Autodesk Inventor part; units mm, degrees
ref_plane "YZ Plane" through (0, 0, 0) normal (1, 0, 0) x (0, 1, 0)
ref_plane "XZ Plane" through (0, 0, 0) normal (0, 1, 0) x (-1, 0, 0)
ref_plane "XY Plane" through (0, 0, 0) normal (0, 0, 1) x (1, 0, 0)
sketch "Sketch1" plane through (0, 0, 0) normal (0, 1, 0) x (-1, 0, 0)
  line L0 (15.8302, -38.0798) -> (-15.7328, -38.1201)
  line L1 (-15.7328, -38.1201) -> (-38.0798, -15.8302)
  line L2 (-38.0798, -15.8302) -> (-38.1201, 15.7328)
  line L3 (-38.1201, 15.7328) -> (-15.8302, 38.0798)
  line L4 (-15.8302, 38.0798) -> (15.7328, 38.1201)
  line L5 (15.7328, 38.1201) -> (38.0798, 15.8302)
  line L6 (38.0798, 15.8302) -> (38.1201, -15.7328)
  line L7 (38.1201, -15.7328) -> (15.8302, -38.0798)
  point P0 (0, 0)
  point P1 (0, 0)
  dimension "d0" = 76.2
extrude "Extrusion1" add sketch "Sketch1" along normal blind 3.175
sketch "Sketch3" plane through (0, 3.175, 0) normal (0, 1, 0) x (1, 0, 0)
  line L0 (38.1201, -15.7328) -> (38.0798, 15.8302)
  line L1 (-38.1201, 15.7328) -> (-38.0798, -15.8302)
  line L2 (32.9198, -20.9465) -> (32.8661, 21.0306)
  line L3 (-32.9198, 20.9465) -> (-32.8661, -21.0306)
  line L4 (-38.1201, 15.7328) -> (-38.0798, -15.8302)
  line L5 (38.1201, -15.7328) -> (38.0798, 15.8302)
  line L6 (38.1201, -15.7328) -> (32.9198, -20.9465)
  line L7 (38.0798, 15.8302) -> (38.1201, -15.7328)
  line L8 (38.1201, -15.7328) -> (38.0798, 15.8302)
  line L9 (38.0798, 15.8302) -> (32.8661, 21.0306)
  line L10 (-32.9198, 20.9465) -> (-38.1201, 15.7328)
  line L11 (-38.1201, 15.7328) -> (-38.0798, -15.8302)
  line L12 (-38.0798, -15.8302) -> (-38.1201, 15.7328)
  line L13 (-38.0798, -15.8302) -> (-32.8661, -21.0306)
  line L14 (-38.0798, -15.8302) -> (-15.7328, -38.1201)
  line L15 (15.8302, -38.0798) -> (38.1201, -15.7328)
  line L16 (38.0798, 15.8302) -> (15.7328, 38.1201)
  line L17 (38.1201, -15.7328) -> (32.9198, -20.9465)
  line L18 (38.0798, 15.8302) -> (32.8661, 21.0306)
  line L19 (15.7328, 38.1201) -> (38.0798, 15.8302)
  line L20 (38.1201, -15.7328) -> (38.0798, 15.8302)
  point P0 (0, 0)
  dimension "d5" = 5.207
  dimension "d6" = 5.207
extrude "Extrusion2" add sketch "Sketch3" along normal blind 35.56
sketch "Sketch5" plane through (38.0798, 0, -15.8302) normal (1, 0, -0.0013) x (-0.0013, 0, -1)
  circle A0 centre (-15.7815, 18.415) radius 11.43
  circle A1 centre (-15.7815, 18.415) radius 11.684
  point P0 (-15.7815, 0)
  dimension "d9" = 0.254
extrude "Extrusion3" cut sketch "Sketch5" against normal blind 26.416 contours A0 | A1
sketch "Sketch6" plane through (-38.0798, 0, 15.8302) normal (-1, 0, 0.0013) x (0.0013, 0, 1)
  circle A0 centre (-15.7815, 18.415) radius 11.43
  circle A1 centre (-15.7815, 18.415) radius 11.684
  point P0 (-15.7815, 0)
  dimension "d12" = 0.254
extrude "Extrusion4" cut sketch "Sketch6" against normal blind 26.416 contours A0 | A1
sketch "Sketch7" plane through (0, 3.175, 0) normal (0, 1, 0) x (1, 0, 0)
  line L0 (15.7328, 38.1201) -> (-15.8302, 38.0798)
  line L1 (20.9465, 32.9198) -> (-21.0306, 32.8661)
  line L2 (-15.8302, 38.0798) -> (-32.9198, 20.9465)
  line L3 (32.8661, 21.0306) -> (15.7328, 38.1201)
  line L4 (-38.1201, 15.7328) -> (-15.8302, 38.0798)
  line L5 (-21.0306, 32.8661) -> (-15.8302, 38.0798)
  line L6 (-15.8302, 38.0798) -> (15.7328, 38.1201)
  line L7 (20.9465, 32.9198) -> (15.7328, 38.1201)
  point P0 (0, 0)
  dimension "d15" = 5.207
extrude "Extrusion5" add sketch "Sketch7" along normal blind 35.56
sketch "Sketch8" plane through (-15.8302, 0, -38.0798) normal (-0.0013, 0, -1) x (-1, 0, 0.0013)
  circle A0 centre (-15.7815, 18.415) radius 11.43
  circle A1 centre (-15.7815, 18.415) radius 11.684
  point P0 (-15.7815, 0)
  dimension "d18" = 0.254
extrude "Extrusion6" cut sketch "Sketch8" against normal blind 26.416 contours A0 | A1
sketch "Sketch9" plane through (0, 3.175, 0) normal (0, 1, 0) x (1, 0, 0)
  line L0 (-9.3728, -20.3542) -> (-9.3647, -26.7042)
  line L1 (8.6353, -26.6812) -> (8.6272, -20.3312)
  line L2 (-8.3634, -27.7029) -> (7.6366, -27.6825)
  line L3 (-9.3728, -20.3542) -> (8.6366, -20.3542)
  line L4 (8.6366, -20.3542) -> (8.6366, -27.6812)
  line L5 (8.6366, -27.6812) -> (-9.3728, -27.6812)
  line L6 (-9.3728, -27.6812) -> (-9.3728, -20.3542)
  point P0 (0, 0)
extrude "Extrusion7" add sketch "Sketch9" along normal blind 26.67
sketch "Sketch10" plane through (0, 29.845, 0) normal (0, 1, 0) x (1, 0, 0)
  arc A0 (-5.3692, -23.1491) -> (-5.3658, -25.8491) centre (-5.3675, -24.4991) ccw
  arc A1 (-5.3658, -25.8491) -> (-5.3692, -23.1491) centre (-5.3675, -24.4991) ccw
  arc A2 (4.6308, -23.1363) -> (4.6342, -25.8363) centre (4.6325, -24.4863) ccw
  arc A3 (4.6342, -25.8363) -> (4.6308, -23.1363) centre (4.6325, -24.4863) ccw
  circle A4 centre (-5.3675, -24.4991) radius 1.016
  circle A5 centre (4.6325, -24.4863) radius 1.016
  point P0 (0, 0)
  dimension "d24" = 1.35
  dimension "d25" = 2.032
  dimension "d26" = 2.032
extrude "Extrusion8" cut sketch "Sketch10" against normal blind 12.7 contours A4 | A5
sketch "Sketch11" plane through (-9.3728, 3.175, 27.6812) normal (0, 0, 1) x (1, 0, 0)
  line L0 (18.0094, 0) -> (0, 0)
  line L1 (5.1947, 6.35) -> (12.8147, 6.35)
  line L2 (12.8147, 6.35) -> (12.8147, 0)
  line L3 (12.8147, 0) -> (5.1947, 0)
  line L4 (5.1947, 0) -> (5.1947, 6.35)
  line L5 (18.0094, 0) -> (18.0094, 26.67)
  point P0 (9.3728, -3.175)
  dimension "d31" = 5.1947
  dimension "d32" = 7.62
  dimension "d33" = 6.35
  dimension "d36" = 0
extrude "Extrusion9" cut sketch "Sketch11" against normal blind 12.7
fillet "Fillet2" radius 3.175 4 edges at (-6.7754, 3.175, 27.6812) (-9.3728, 3.175, 24.0177) (6.0392, 3.175, 27.6812) (8.6366, 3.175, 24.0177)
properties part number "Main_assy_base"
For this review, take the finished solid that the model builds, in its own axes (mm). Give positions to 0.01 mm unless a question says otherwise; leave off trailing zeros. Order: outer loops, then holes, each group sorted by start corner. A loop starts at its lowest first (then second) coordinate and runs counter-clockwise, first axis right, second up. Notation, with made-up numbers: (-14.75, 21) -> (23.25, 21) arc R26 cw to (23.25, 59) -> close; hole circle Ø7 at (30.5, -21.5). An arc over 180 degrees is marked (long way). Write item = value, one per line.
1) We need section C-C, the plane y = 36.5. Give the boundary of the cut face in (x, z).
Findings:
outline = (-38.12, -15.73) -> (-32.92, -20.95) -> (-32.87, 21.03) -> (-38.08, 15.83) -> close; (-21.03, -32.87) -> (-15.83, -38.08) -> (15.73, -38.12) -> (20.95, -32.92) -> close; (32.87, -21.03) -> (38.08, -15.83) -> (38.12, 15.73) -> (32.92, 20.95) -> close
2) Insertion check: pin 1 (8 mm diameter, centred on x = 1, z = 25, fed in from +Y) (3 decimals); pin 2 (1.6 mm diameter, centred on x = 4.5, z = 24.5, fed in from +Y) (3 decimals); pin 3 (5 mm diameter, centred on y = 6, z = 27, fed in from -X); pin 4 (3 mm diameter, centred on x = 24, y = 5, fed in from -Z). Each pin has a flat end and moves straight along its axis. Give the tip position at first contact, or say it passes through.
Findings:
pin_1 = 29.845
pin_2 = 17.145
pin_3 = -11.15
pin_4 = through
3) To check wall thickness, follow L1, parallel to X at y = 34, z = 9; L2, parallel to Y at x = -2.5, z = 21.5 (3 decimals); L3, parallel to Y at x = -33, z = 0 (3 decimals). State the ranges of each line that lie inside material, in increasing order. Write a range as from..to.
Findings:
L1 = -38.09..-32.88, 32.9..38.11
L2 = 0..3.175, 9.525..29.845
L3 = 0..6.731, 30.099..38.735
4) Draft analysis for pull direction Z (two halves, no side actions). For faces 1 (the face through (-35.48, 20.71, -18.38)), 2 (the face through (5, 17.145, 24)), 3 (the face through (0, 29.845, 24)), state which applies: pulls with the +Z half, pulls with the -Z half, needs draft (parallel to the pull), parting line crosses it, or undercut.
Findings:
face_1 = pulls with the -Z half
face_2 = undercut
face_3 = needs draft
5) We need section B-B, the plane x = 19. Give the boundary of the cut face in (y, z) (3 decimals), and give its area (3 significant figures).
Findings:
outline = (0, -34.861) -> (38.735, -34.861) -> (38.735, -32.917) -> (3.175, -32.917) -> (3.175, 34.902) -> (0, 34.902) -> close
area = 291 mm^2
6) We need section A-A, the plane y = 10.5. Give the boundary of the cut face in (x, z).
Findings:
outline = (-38.12, -15.73) -> (-32.92, -20.95) -> (-32.9, -8.55) -> (-38.11, -8.55) -> close; (-38.09, 8.64) -> (-32.88, 8.64) -> (-32.87, 21.03) -> (-38.08, 15.83) -> close; (-21.03, -32.87) -> (-15.83, -38.08) -> (-8.64, -38.09) -> (-8.64, -32.88) -> close; (-9.37, 20.35) -> (8.64, 20.35) -> (8.64, 27.68) -> (-9.37, 27.68) -> close; (8.55, -38.11) -> (15.73, -38.12) -> (20.95, -32.92) -> (8.55, -32.9) -> close; (32.87, -21.03) -> (38.08, -15.83) -> (38.09, -8.64) -> (32.88, -8.64) -> close; (32.9, 8.55) -> (38.11, 8.55) -> (38.12, 15.73) -> (32.92, 20.95) -> close
7) We need section D-D, the plane z = -14.5. Give the boundary of the cut face in (x, y) (1 decimal), and give its area (3 significant figures).
Findings:
outline = (-38.1, 0) -> (38.1, 0) -> (38.1, 38.7) -> (32.9, 38.7) -> (32.9, 3.2) -> (-32.9, 3.2) -> (-32.9, 38.7) -> (-38.1, 38.7) -> close
area = 612 mm^2
